Read the model definition and answer for the solid it produces. Units are mm, in the model's axes. Face numbers are marked on the shaded views. A direction names the side the tool comes from. Coordinates: 2 decimals unless noted, no trailing zeros. Order: outer loops, then holes, each group sorted by start corner. A loop starts at its lowest first (then second) coordinate and runs counter-clockwise, first axis right, second up.
```python
from build123d import *

# Parameters (mm, degrees)
F0_W     = 990.6
F0_H     = 711.2
F1_DEPTH = 990.6
F2_W     = 990.6
F2_H     = 114.3
F3_DEPTH = 685.8
F2_H_2   = 800.1
F2_W_2   = 485.775
F2_H_3   = 628.65
F2_H_4   = 152.4
F4_DEPTH = 6.35
F2_H_5   = 76.2
F5_DEPTH = 76.2
F2_W_3   = 152.4
F2_H_6   = 12.7
F2_W_4   = 12.7
F6_DEPTH = 19.05
F7_W     = 838.2
F7_H     = 482.6
F8_DEPTH = 787.4


with BuildPart() as f1:
    # F0 (on Top) → F1 (new body)
    with BuildSketch(Plane.XY):
        Rectangle(F0_W, F0_H)
    extrude(amount=F1_DEPTH)

    # F2 (on face) → F3 (cut)
    with BuildSketch(Plane.XZ.offset(355.6)):
        with Locations((0, 933.45)):
            Rectangle(F2_W, F2_H)
    extrude(amount=-F3_DEPTH, mode=Mode.SUBTRACT)

    # F2 (on face) → F4 (cut)
    with BuildSketch(Plane.XZ.offset(355.6)):
        with Locations((0, 476.25)):
            Rectangle(F2_W, F2_H_2)
        with Locations((-246.0625, 396.875)):
            Rectangle(F2_W_2, F2_H_3, mode=Mode.SUBTRACT)
        with Locations((246.0625, 396.875)):
            Rectangle(F2_W_2, F2_H_3, mode=Mode.SUBTRACT)
        with Locations((-246.0625, 793.75)):
            Rectangle(F2_W_2, F2_H_4, mode=Mode.SUBTRACT)
        with Locations((246.0625, 793.75)):
            Rectangle(F2_W_2, F2_H_4, mode=Mode.SUBTRACT)
    extrude(amount=-F4_DEPTH, mode=Mode.SUBTRACT)

    # F2 (on face) → F5 (cut)
    with BuildSketch(Plane.XZ.offset(355.6)):
        with Locations((0, 38.1)):
            Rectangle(F2_W, F2_H_5)
    extrude(amount=-F5_DEPTH, mode=Mode.SUBTRACT)

    # F2 (on face) → F6 (join)
    with BuildSketch(Plane.XZ.offset(355.6)):
        with Locations((-246.0625, 793.75)):
            Rectangle(F2_W_3, F2_H_6)
        with Locations((246.0625, 793.75)):
            Rectangle(F2_W_3, F2_H_6)
        with Locations((60.325, 396.875)):
            Rectangle(F2_W_4, F2_H_4)
        with Locations((-60.325, 396.875)):
            Rectangle(F2_W_4, F2_H_4)
    extrude(amount=F6_DEPTH)

    # F7 (on face) → F8 (cut)
    with BuildSketch(Plane(origin=(0, 0, 0), x_dir=(1, 0, 0), z_dir=(0, 0, -1))):
        with Locations((0, -38.1)):
            Rectangle(F7_W, F7_H)
    extrude(amount=-F8_DEPTH, mode=Mode.SUBTRACT)


solid = f1.part
```
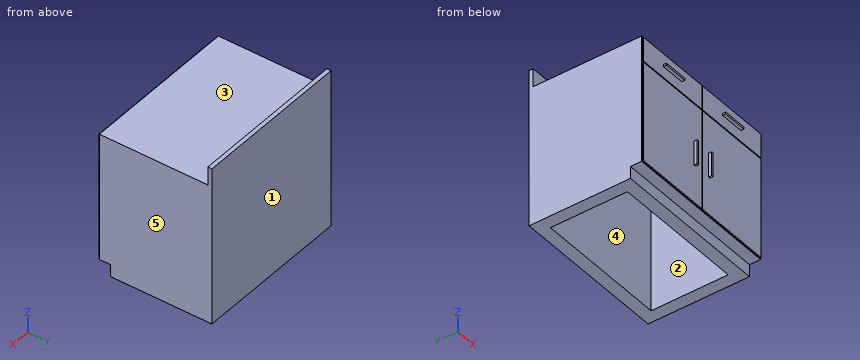
1) A cutting plane is placed at A-A, the plane z = 377.5. Determine the outline of the cut face in (x, y) (3 decimals), and give its area (3 significant figures).
A:
outline: (-495.3, -349.25) - (-488.95, -349.25) - (-488.95, -355.6) - (-66.675, -355.6) - (-66.675, -374.65) - (-53.975, -374.65) - (-53.975, -355.6) - (-3.175, -355.6) - (-3.175, -349.25) - (3.175, -349.25) - (3.175, -355.6) - (53.975, -355.6) - (53.975, -374.65) - (66.675, -374.65) - (66.675, -355.6) - (488.95, -355.6) - (488.95, -349.25) - (495.3, -349.25) - (495.3, 355.6) - (-495.3, 355.6) - close; hole (-419.1, -203.2) - (419.1, -203.2) - (419.1, 279.4) - (-419.1, 279.4) - close
area: 300,000 mm2
2) Which of the six approach directions +Z, -Z, +X, -X, +Y, -Y give full straight-line access (tool end or side, diameter ignored) to the marked faces 4 and 5?
A:
face 4: -Z
face 5: +Z, -Z, +X, +Y, -Y
3) A cutting plane is placed at B-B, the plane y = -75.5. Determine the outline of the cut face in (x, z).
A:
outline: (-495.3, 0) - (-419.1, 0) - (-419.1, 787.4) - (419.1, 787.4) - (419.1, 0) - (495.3, 0) - (495.3, 876.3) - (-495.3, 876.3) - close
4) Straight lines are drawn through the part: line 1 (Y direction, x = 402, z = 519); line 2 (X direction, y = 200.5, z = 502); line 3 (Y direction, x = -2.5, z = 519). For each, find the intervals that lie inside material, in ascending order.
A:
line 1: y = -355.6 to -203.2, 279.4 to 355.6
line 2: x = -495.3 to -419.1, 419.1 to 495.3
line 3: y = -349.25 to -203.2, 279.4 to 355.6
5) A cutting plane is placed at D-D, the plane z = 106.5. Determine the outline of the cut face in (x, y) (3 decimals).
A:
outline: (-495.3, -349.25) - (-488.95, -349.25) - (-488.95, -355.6) - (-3.175, -355.6) - (-3.175, -349.25) - (3.175, -349.25) - (3.175, -355.6) - (488.95, -355.6) - (488.95, -349.25) - (495.3, -349.25) - (495.3, 355.6) - (-495.3, 355.6) - close; hole (-419.1, -203.2) - (419.1, -203.2) - (419.1, 279.4) - (-419.1, 279.4) - close
6) Determine the mould class of the marked faces 1, 2 and 3 for opening direction Y: pulls with the +Y half, pulls with the -Y half, needs draft (parallel to the pull), parting line crosses it, or undercut.
A:
face 1: pulls with the +Y half
face 2: undercut
face 3: needs draft
7) A cutting plane is placed at C-C, the plane x = 190. Determine the outline of the cut face in (y, z).
A:
outline: (-374.65, 787.4) - (-355.6, 787.4) - (-355.6, 717.55) - (-349.25, 717.55) - (-349.25, 711.2) - (-355.6, 711.2) - (-355.6, 82.55) - (-349.25, 82.55) - (-349.25, 76.2) - (-279.4, 76.2) - (-279.4, 0) - (-203.2, 0) - (-203.2, 787.4) - (279.4, 787.4) - (279.4, 0) - (355.6, 0) - (355.6, 990.6) - (330.2, 990.6) - (330.2, 876.3) - (-349.25, 876.3) - (-349.25, 869.95) - (-355.6, 869.95) - (-355.6, 800.1) - (-374.65, 800.1) - close
8) Flat-ended cylindrical pins translate along their axes: pin 1 Ø6 at (x, z) = (339, 881) entering from -Y; pin 2 Ø6 at (x, y) = (-88, 43.5) entering from -Z; pin 3 Ø5 at (x, z) = (-137.5, 360.5) entering from -Y. Find the tip coordinate at first contact, or state that the pin passes through.
A:
pin 1: stops at y = 330.2
pin 2: stops at z = 787.4
pin 3: stops at y = -355.6
